CAD build for the part. Positions are in the model's coordinates, mm. A direction names the side the tool comes from. Round coordinates to 2 decimals unless told otherwise and drop trailing zeros. Loops run counter-clockwise (first coordinate to the right, second up) from the corner with the lowest first, then second, coordinate; pieces in that order, holes last.
Autodesk Inventor part; units mm, degrees
ref_plane "YZ Plane" through (0, 0, 0) normal (1, 0, 0) x (0, 1, 0)
ref_plane "XZ Plane" through (0, 0, 0) normal (0, 1, 0) x (-1, 0, 0)
ref_plane "XY Plane" through (0, 0, 0) normal (0, 0, 1) x (1, 0, 0)
sketch "Sketch1" plane through (0, 0, 0) normal (0, 1, 0) x (-1, 0, 0)
  line L0 (30.1625, 30.1625) -> (-30.1625, 30.1625)
  line L1 (-30.1625, 30.1625) -> (-30.1625, -30.1625)
  line L2 (-30.1625, -30.1625) -> (30.1625, -30.1625)
  line L3 (30.1625, -30.1625) -> (30.1625, 30.1625)
  circle A0 centre (0, 0) radius 33.3375 construction
  circle A1 centre (0, 0) radius 28.575
  line L4 (-30.1625, 30.1625) -> (30.1625, -30.1625) construction
  line L5 (30.1625, 30.1625) -> (-30.1625, -30.1625) construction
  circle A2 centre (23.5732, 23.5732) radius 2.159
  circle A3 centre (23.5732, -23.5732) radius 2.159
  circle A4 centre (-23.5732, 23.5732) radius 2.159
  circle A5 centre (-23.5732, -23.5732) radius 2.159
  point P0 (0, 0)
  point P1 (0, 0)
  dimension "d0" = 60.325
  dimension "d1" = 60.325
  dimension "d2" = 66.675
  dimension "d3" = 57.15
  dimension "d4" = 4.318
  dimension "d5" = 4.318
  dimension "d6" = 4.318
  dimension "d7" = 4.318
extrude "Extrusion1" add sketch "Sketch1" along normal blind 3.175 contours L3 L2 L1 L0 | A1
sketch "Sketch2" plane through (0, 3.175, 0) normal (0, 1, 0) x (1, 0, 0)
  circle A0 centre (0, 0) radius 27.94
  circle A1 centre (0, 0) radius 28.575 construction
  point P0 (0, 0)
  dimension "d10" = 55.88
  dimension "d17" = 57.15
extrude "Extrusion2" add sketch "Sketch2" along normal blind 1.905
fillet "Fillet1" radius 3.175 4 edges at (30.1625, 1.5875, 30.1625) (-30.1625, 1.5875, 30.1625) (30.1625, 1.5875, -30.1625) (-30.1625, 1.5875, -30.1625)
sketch "Sketch3" plane through (0, 5.08, 0) normal (0, 1, 0) x (1, 0, 0)
  line L0 (-12.7, -1.8506) -> (12.7, -1.8506)
  line L1 (12.7, -1.8506) -> (12.7, 23.5494)
  line L2 (12.7, 23.5494) -> (-12.7, 23.5494)
  line L3 (-12.7, 23.5494) -> (-12.7, -1.8506)
  circle A0 centre (0, 0) radius 27.94
  circle A1 centre (0, 0) radius 27.94 construction
  circle A2 centre (0.0007, -17.939) radius 5.08
  line L4 (16.9084, 0) -> (27.94, 0) construction
  circle A3 centre (22.4242, 0) radius 3.302
  circle A4 centre (0.0007, -17.939) radius 9.017
  line L5 (-12.7, 23.5494) -> (12.7, 23.5494)
  line L6 (12.7, 23.5494) -> (12.7, 27.3594)
  line L7 (12.7, 27.3594) -> (-12.7, 27.3594)
  line L8 (-12.7, 27.3594) -> (-12.7, 23.5494)
  line L9 (-12.7, -1.8506) -> (12.7, -1.8506)
  line L10 (12.7, -1.8506) -> (12.7, -5.6606)
  line L11 (12.7, -5.6606) -> (-12.7, -5.6606)
  line L12 (-12.7, -5.6606) -> (-12.7, -1.8506)
  circle A5 centre (0, 0) radius 27.94 construction
  line L13 (9.7799, 26.1725) -> (9.7799, -5.6606) construction
  line L14 (-10.16, 27.3594) -> (-10.16, -5.6606) construction
  circle A6 centre (22.4242, 0) radius 5.08 construction
  line L15 (-18.288, 29.1374) -> (18.288, 29.1374) construction
  line L16 (18.288, 29.1374) -> (18.288, -7.4386) construction
  line L17 (18.288, -7.4386) -> (-18.288, -7.4386) construction
  line L18 (-18.288, -7.4386) -> (-18.288, 29.1374) construction
  line L19 (-18.288, 29.1374) -> (18.288, -7.4386) construction
  line L20 (18.288, 29.1374) -> (-18.288, -7.4386) construction
  line L21 (18.9952, 6.35) -> (25.8532, 6.35) construction
  line L22 (25.8532, 6.35) -> (25.8532, -6.35) construction
  line L23 (25.8532, -6.35) -> (18.9952, -6.35) construction
  line L24 (18.9952, -6.35) -> (18.9952, 6.35) construction
  line L25 (18.9952, 6.35) -> (25.8532, -6.35) construction
  line L26 (25.8532, 6.35) -> (18.9952, -6.35) construction
  circle A7 centre (0.0007, -17.939) radius 9.525 construction
  point P0 (0, 10.8494)
  dimension "d18" = 25.4
  dimension "d19" = 25.4
  dimension "d32" = 10.16
  dimension "d33" = 6.604
  dimension "d34" = 18.034
  dimension "d37" = 3.81
  dimension "d38" = 3.81
  dimension "d48" = 10.16
  dimension "d49" = 36.576
  dimension "d50" = 36.576
  dimension "d51" = 6.858
  dimension "d52" = 12.7
  dimension "d53" = 19.05
extrude "Extrusion4" cut sketch "Sketch3" against normal through all contours L3 L2 L1 L0 | A2 | A3
extrude "Extrusion5" cut sketch "Sketch3" against normal blind 2.54 contours A4
extrude "Extrusion6" add sketch "Sketch3" against normal blind 11.811 separate body contours L0 L10 L11 L12 | L8 A0 L7 L6 L2 | L8 L7 A0 | A0 L7 L6
sketch "Sketch4" plane through (-12.7, 5.08, 5.6606) normal (0, 0, 1) x (1, 0, 0)
  line L0 (25.4, -8.255) -> (0, -8.255) construction
  line L1 (25.4, 0) -> (25.4, -11.811) construction
  line L2 (0, 0) -> (0, -11.811) construction
  point P0 (12.7, -5.08)
  point P1 (2.5418, -8.255)
  point P2 (22.8582, -8.255)
hole "Hole1" at (10.1582, -3.175, 5.6606) at (-10.1582, -3.175, 5.6606) direction (0, 0, -1) diameter 2.032 end through all bodies 2
combine bodies "Combine1" operation type add bodies to combine 1 2
delete faces "Delete1" heal yes whole lump no faces at (10.3555, 4.445, -27.3594) (-8.0109, 4.445, -27.3594) (12.7, 3.81, -26.5352) (-12.7, 3.81, -25.711)
properties part number "icarus-sam-instrument-mount"
Item 1: Cut at C-C, the plane x = 0. Give the cut face in (y, z) (1 decimal), plus the area to 3 significant figures.
Answers follow:
outline: (-6.7, -27.4) - (0, -27.4) - (0, -30.2) - (3.2, -30.2) - (3.2, -27.9) - (5.1, -27.9) - (5.1, -23.5) - (-6.7, -23.5) - close; (-6.7, 1.9) - (5.1, 1.9) - (5.1, 8.9) - (2.5, 8.9) - (2.5, 12.9) - (0, 12.9) - (0, 5.7) - (-6.7, 5.7) - close; (0, 23) - (2.5, 23) - (2.5, 27) - (5.1, 27) - (5.1, 27.9) - (3.2, 27.9) - (3.2, 30.2) - (0, 30.2) - close
area: 149 mm2
Item 2: Two-plate mould, pull along X, no slides. Class faces 1 (the cylindrical face through (2.441, 4.114, -27.833)), 2 (the cylindrical face through (25.287, 1.565, -22.259)), 3 (the cylindrical face through (29.208, 1.61, 29.257)): released by +X, released by -X, zero draft, split by the parting line, or undercut.
Answers follow:
face 1: split by the parting line
face 2: undercut
face 3: released by +X
Item 3: 3-axis set-ups, long thin cutter, end or side, ignore diameter. For faces 4 (the flat face through (-12.7, -3, 4)), 5 (the flat face through (12.7, 3, -11)), 6 (the cylindrical face through (-1.17, 3.83, 9)): which of +Z, -Z, +X, -X, +Y, -Y reach the whole face in a straight line?
Answers follow:
face 4: +Z, -Z, -X, -Y
face 5: +Y, -Y
face 6: +Y
Item 4: Cut at A-A, the plane y = -5.75. Give the cut face in (x, z).
Answers follow:
outline: (-12.7, -27.36) - (12.7, -27.36) - (12.7, -23.55) - (-12.7, -23.55) - close; (-12.7, 1.85) - (12.7, 1.85) - (12.7, 5.66) - (-12.7, 5.66) - close
Item 5: Probe line 1 (X direction, y = 1.25, z = -21); line 2 (X direction, y = 1.25, z = -3); line 3 (X direction, y = -1.5, z = -26). List the from-to ranges inside material, lowest first.
Answers follow:
line 1: x = -30.16 to -12.7, 12.7 to 30.16
line 2: x = -30.16 to -12.7, 12.7 to 21.04, 23.8 to 30.16
line 3: x = -12.7 to 12.7
Item 6: Flat gauge pins, fed straight in: P1, Ø2.5, axis at x = -10.16, y = -3.18, coming from the +Z side; P2, Ø4, axis at x = 22.42, z = 0, coming from the -Y side; P3, Ø1, axis at x = -21.5, z = -19, coming from the +Y side (3 decimals); P4, Ø1.9, axis at y = -5, z = -25.5, coming from the -X side. Where does each tip first touch, or does it go through?
Answers follow:
P1: stops at z = 5.66
P2: passes through
P3: stops at y = 3.175
P4: stops at x = -12.7
Item 7: Cut at D-D, the plane x = 7.5. Give the cut face in (y, z) (1 decimal).
Answers follow:
outline: (-6.7, -27.4) - (0, -27.4) - (0, -30.2) - (3.2, -30.2) - (3.2, -26.9) - (5.1, -26.9) - (5.1, -23.5) - (-6.7, -23.5) - close; (-6.7, 1.9) - (5.1, 1.9) - (5.1, 12.9) - (2.5, 12.9) - (2.5, 22.9) - (5.1, 22.9) - (5.1, 26.9) - (3.2, 26.9) - (3.2, 30.2) - (0, 30.2) - (0, 5.7) - (-6.7, 5.7) - close
Item 8: Cut at B-B, the plane z = 0. Give the cut face in (x, y) (1 decimal), plus the area to 3 significant figures.
Answers follow:
outline: (-30.2, 0) - (-12.7, 0) - (-12.7, 5.1) - (-27.9, 5.1) - (-27.9, 3.2) - (-30.2, 3.2) - close; (12.7, 0) - (19.1, 0) - (19.1, 5.1) - (12.7, 5.1) - close; (25.7, 0) - (30.2, 0) - (30.2, 3.2) - (27.9, 3.2) - (27.9, 5.1) - (25.7, 5.1) - close
area: 135 mm2
